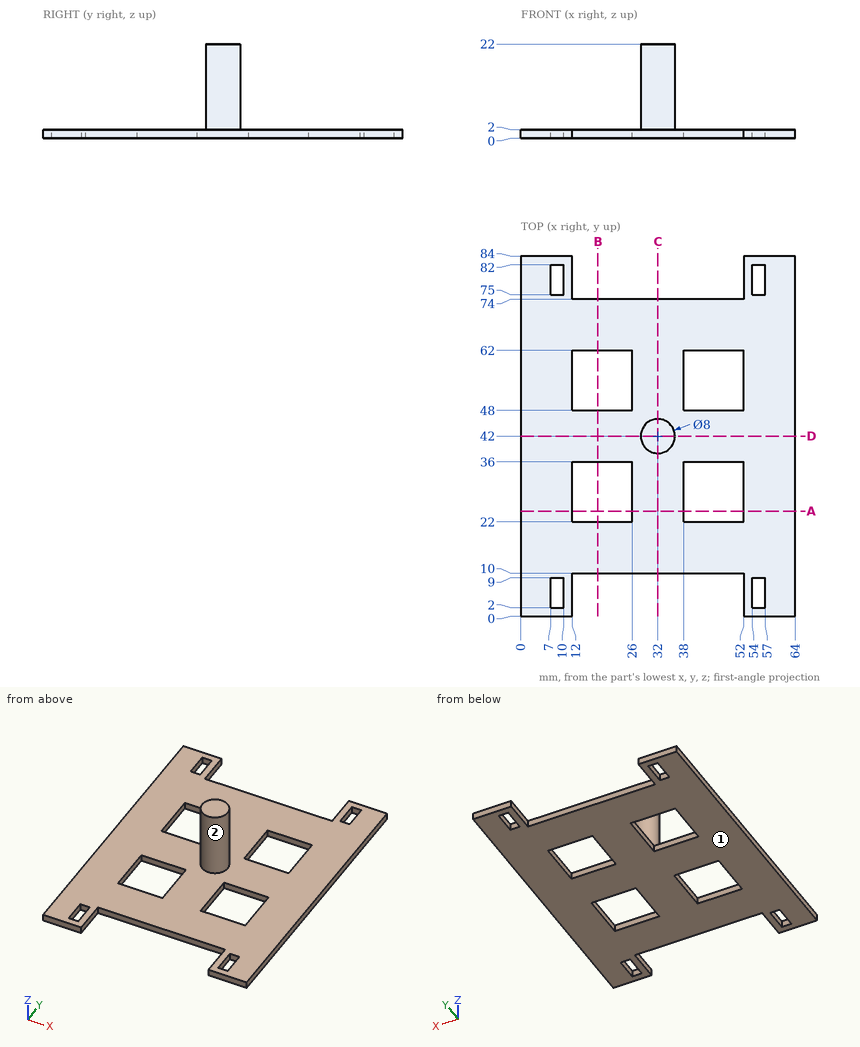
Job drawing, mm, ordinate dimensions from the low corner. One solid piece. A direction names the side the tool comes from. Coordinates: 2 decimals unless noted, no trailing zeros. Order: outer loops, then holes, each group sorted by start corner. A loop starts at its lowest first (then second) coordinate and runs counter-clockwise, first axis right, second up. Notation, with made-up numbers: (33.25, 44) -> (54.25, 44) arc R23 ccw to (54.25, 69) -> close; hole circle Ø11 at (50, 82.25). An arc over 180 degrees is marked (long way). Put each result on its own line as item: value. Start each with the question number.
(1) Band-saw the part on C-C (x = 32). Give the cut face in (y, z).
(2) Probe line 1 along Z through (x, y) = (3.5, 28.5); line 2 along Y through (x, z) = (32, 8.5); line 3 along X through (y, z) = (43, 5). List the from-to ranges inside material, lowest first. Write a range as [from, to].
(3) Band-saw the part on B-B (x = 18). Give the cut face in (y, z), then the cut area to 3 significant figures.
(4) Band-saw the part on D-D (y = 42). Give the cut face in (x, z).
(5) Pin check, flat tips, straight feed: pin 1 Ø0.6 at (x, z) = (9, 0.5) entering from -Y; pin 2 Ø1.6 at (x, z) = (48, 0.5) entering from +Y; pin 3 Ø0.6 at (x, z) = (42.5, 1) entering from -Y; pin 4 Ø6 at (x, y) = (49, 73.5) entering from +Z. Stop position of each tip, or through.
(6) Band-saw the part on A-A (y = 24.5). Give the cut face in (x, z).
(7) Which spindle directions (+Z, -Z, +X, -X, +Y, -Y) get a long thin tool onto all of the face, cutting with end or side? Do the marked faces 1 and 2. Say none if no direction does.
Determined:
1. outline: (10, 0) -> (74, 0) -> (74, 2) -> (46, 2) -> (46, 22) -> (38, 22) -> (38, 2) -> (10, 2) -> close
2. line 1: z = [0, 2]
2. line 2: y = [38, 46]
2. line 3: x = [28.13, 35.87]
3. outline: (10, 0) -> (22, 0) -> (22, 2) -> (10, 2) -> close; (36, 0) -> (48, 0) -> (48, 2) -> (36, 2) -> close; (62, 0) -> (74, 0) -> (74, 2) -> (62, 2) -> close
3. area: 72.0 mm²
4. outline: (0, 0) -> (64, 0) -> (64, 2) -> (36, 2) -> (36, 22) -> (28, 22) -> (28, 2) -> (0, 2) -> close
5. pin 1: stops at y = 0
5. pin 2: stops at y = 74
5. pin 3: stops at y = 10
5. pin 4: stops at z = 2
6. outline: (0, 0) -> (12, 0) -> (12, 2) -> (0, 2) -> close; (26, 0) -> (38, 0) -> (38, 2) -> (26, 2) -> close; (52, 0) -> (64, 0) -> (64, 2) -> (52, 2) -> close
7. face 1: -Z, +X, -X, +Y, -Y
7. face 2: +Z
